Part print with two shaded views. Sizes in mm from the minimum x, y, z corner. A direction names the side the tool comes from. Give positions to 0.01 mm unless a question says otherwise; leave off trailing zeros. Write each loop counter-clockwise with the first axis right and the second up, starting at its lowest first coordinate (ties: lowest second). Pieces come first, ordered by that corner, then holes.
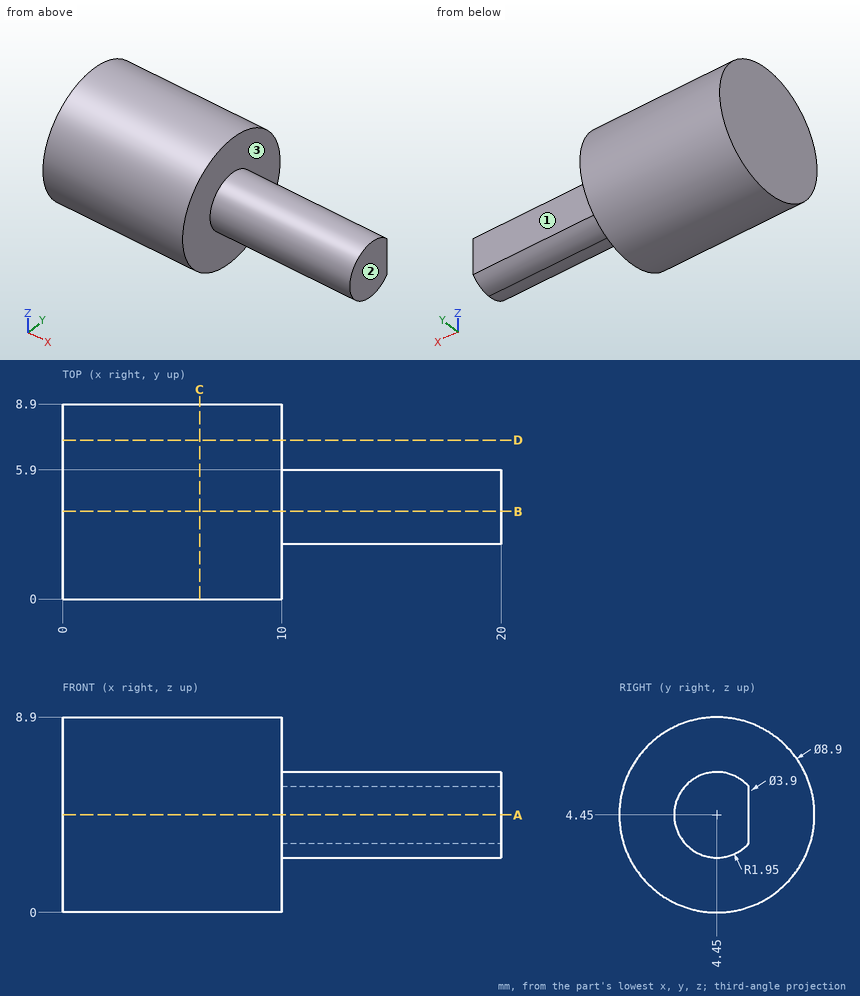
(1) Drop flat-ended pins along their axis: pin 1 (2 mm diameter, centred on x = 15.5, z = 5, fed in from +Y); pin 2 (3 mm diameter, centred on y = 7.5, z = 6.5, fed in from +X); pin 3 (3 mm diameter, centred on x = 16.5, z = 2.5, fed in from -Y). Give the stop position or say it passes through.
(2) Saw through at B-B, the plane y = 4. List the corners of the cut face in (x, z), plus the area to 3 significant figures.
(3) Saw through at C-C, the plane x = 6.25. List the corners of the cut face in (y, z), plus the area to 3 significant figures.
(4) Saw through at D-D, the plane y = 7.25. List the corners of the cut face in (x, z), plus the area to 3 significant figures.
(5) Probe line 1 (X direction, y = 1.25, z = 4); line 2 (Y direction, x = 11.5, z = 4); line 3 (Y direction, x = 8, z = 2.75). List the from-to ranges inside material, lowest first.
(6) 3-axis set-ups, long thin cutter, end or side, ignore diameter. For the marked faces 1, 2 and 3: which of +Z, -Z, +X, -X, +Y, -Y reach the whole face in a straight line?
(7) Saw through at A-A, the plane z = 4.45. List the corners of the cut face in (x, y).
Computed values:
1. pin 1: stops at y = 5.9
1. pin 2: stops at x = 10
1. pin 3: stops at y = 2.55
2. outline: (0, 0.02) - (10, 0.02) - (10, 2.55) - (20, 2.55) - (20, 6.35) - (10, 6.35) - (10, 8.88) - (0, 8.88) - close
2. area: 126 mm2
3. outline: circle Ø8.9 at (4.45, 4.45)
3. area: 62.2 mm2
4. outline: (0, 0.99) - (10, 0.99) - (10, 7.91) - (0, 7.91) - close
4. area: 69.2 mm2
5. line 1: x = 0 to 10
5. line 2: y = 2.55 to 5.9
5. line 3: y = 0.34 to 8.56
6. face 1: +Z, -Z, +X, +Y
6. face 2: +Z, -Z, +X, +Y, -Y
6. face 3: +X
7. outline: (0, 0) - (10, 0) - (10, 2.5) - (20, 2.5) - (20, 5.9) - (10, 5.9) - (10, 8.9) - (0, 8.9) - close
